Autodesk Inventor part; units mm, degrees
ref_plane "YZ Plane" through (0, 0, 0) normal (1, 0, 0) x (0, 1, 0)
ref_plane "XZ Plane" through (0, 0, 0) normal (0, 1, 0) x (-1, 0, 0)
ref_plane "XY Plane" through (0, 0, 0) normal (0, 0, 1) x (1, 0, 0)
sketch "Boceto1" plane through (0, 0, 0) normal (0, 0, 1) x (1, 0, 0)
  point P0 (0, 0)
sketch "Boceto2" plane through (0, 0, 0) normal (0, 0, 1) x (1, 0, 0)
  line L0 (0, 0) -> (0, 100)
  line L1 (30, 130) -> (30, 130)
  line L2 (60, 100) -> (60, 0)
  line L3 (60, 0) -> (0, 0)
  arc A0 (30, 130) -> (0, 100) centre (30, 100) ccw
  arc A1 (60, 100) -> (30, 130) centre (30, 100) ccw
  point P0 (0, 130)
  point P1 (60, 130)
  dimension "d1" = 30
  dimension "d2" = 100
  dimension "d3" = 60
extrude "Extrusión1" add sketch "Boceto2" along normal mid plane 25
sketch "Boceto9" plane through (0, 0, 12.5) normal (0, -1, 0) x (1, 0, 0)
  circle A0 centre (50, -12.5) radius 4
  line L0 (60, -25) -> (0, -25)
  circle A1 centre (10, -12.5) radius 4
  line L1 (0, -12.5) -> (60, -12.5) construction
  line L2 (60, 0) -> (60, -25) construction
  dimension "d52" = 8
  dimension "d88" = 10
  dimension "d89" = 10
hole "Agujero4" at (10, 0, 0) at (50, 0, 0) direction (0, 1, 0) diameter 8 depth 25
thread "Rosca3"
thread "Rosca4"
sketch "Boceto10" plane through (0, 0, 12.5) normal (0, 0, 1) x (1, 0, 0)
  circle A0 centre (30, 100) radius 11
  circle A1 centre (30, 100) radius 13.0125
  line L0 (60, 0) -> (60, 100)
  line L1 (0, 100) -> (0, 0)
  line L2 (40, 144.843) -> (20, 144.843)
  dimension "d64" = 22
  dimension "d65" = 30
  dimension "d68" = 26.025
  dimension "d90" = 100
extrude "Extrusión5" cut sketch "Boceto10" against normal through all contours A0
extrude "Extrusión6" cut sketch "Boceto10" against normal blind 9
sketch "Boceto12" plane through (0, 0, 12.5) normal (0, 0, 1) x (1, 0, 0)
  line L0 (5, 21.5) -> (15, 21.5)
  line L1 (17, 19.5) -> (17, 17)
  line L2 (15, 15) -> (5, 15)
  line L3 (3, 17) -> (3, 19.5)
  line L4 (45, 21.5) -> (55, 21.5)
  line L5 (57, 19.5) -> (57, 17)
  line L6 (55, 15) -> (45, 15)
  line L7 (43, 17) -> (43, 19.5)
  line L8 (0, 0) -> (60, 0)
  line L9 (10, 0) -> (10, 43.0314) construction
  line L10 (54, 0) -> (46, 0) construction
  line L11 (50, 0) -> (50, 39.0292) construction
  arc A0 (5, 21.5) -> (3, 19.5) centre (5, 19.5) ccw
  arc A1 (3, 17) -> (5, 15) centre (5, 17) ccw
  arc A2 (15, 15) -> (17, 17) centre (15, 17) ccw
  arc A3 (17, 19.5) -> (15, 21.5) centre (15, 19.5) ccw
  arc A4 (45, 21.5) -> (43, 19.5) centre (45, 19.5) ccw
  arc A5 (43, 17) -> (45, 15) centre (45, 17) ccw
  arc A6 (57, 19.5) -> (55, 21.5) centre (55, 19.5) ccw
  arc A7 (55, 15) -> (57, 17) centre (55, 17) ccw
  point P0 (17, 15)
  point P1 (17, 21.5)
  point P2 (3, 15)
  point P3 (43, 21.5)
  point P4 (57, 15)
  point P5 (43, 15)
  dimension "d91" = 14
  dimension "d92" = 14
  dimension "d93" = 6.5
  dimension "d94" = 15
  dimension "d95" = 40
  dimension "d96" = 7
  dimension "d97" = 7
  dimension "d98" = 2
  dimension "d99" = 2
  dimension "d100" = 2
  dimension "d101" = 2
  dimension "d102" = 2
  dimension "d103" = 2
  dimension "d104" = 2
  dimension "d105" = 2
extrude "Extrusión7" cut sketch "Boceto12" against normal blind 20
sketch "Boceto13" plane through (0, 0, 12.5) normal (0, 0, 1) x (1, 0, 0)
  circle A0 centre (30, 20) radius 6
  line L0 (0, 0) -> (60, 0) construction
  line L1 (30, 0) -> (30, 20) construction
  dimension "d108" = 20
  dimension "d109" = 12
extrude "Extrusión8" cut sketch "Boceto13" against normal through all
equation "\"Radio_pliegue\" = Grosor"
equation "\"Anchura_desahogo_plegado\" = Grosor"
equation "\"Profundidad_desahogo_plegado\" = 0.5 * Grosor"
equation "\"Tamaño_destalonado\" = 4 * Grosor"
equation "\"Remanente_mínimo\" = 2 * Grosor"
equation "\"Radiodetransición\" = Radio_pliegue"
equation "\"Tamaño_de_radio_de_Jacobi\" = Grosor"
equation "\"TamañoSeparación\" = Grosor"
properties part number "soporte_riel" material "Nilón 6/6"
For this review, take the finished solid that the model builds, in its own axes (mm). A direction names the side the tool comes from. Give positions to 0.01 mm unless a question says otherwise; leave off trailing zeros. Loops run counter-clockwise (first coordinate to the right, second up) from the corner with the lowest first, then second, coordinate; pieces in that order, holes last.
Item 1: Draft analysis for pull direction X (two halves, no side actions). For faces 1 (the flat face through (30, 0, 0)), 2 (the flat face through (50, 25, 0)), 3 (the flat face through (0, 49, 0)), state which applies: +X half, -X half, draft (parallel to the pull), parting line (faces both ways), or undercut.
Item 2: Take a section at D-D, the plane y = 98. State the section outline as (x, z) points, and give its area (3 significant figures).
Item 3: Take a section at C-C, the plane x = 21.5. State the section outline as (y, z) points.
Item 4: Tool access review of faces 4 (the cylindrical face through (13.905, 7.605, 0.867)), 5 (the flat face through (17, 18, 3)), 6 (the cylindrical face through (28.568, 110.906, -4.388)): name each direction out of +Z, -Z, +X, -X, +Y, -Y from which nothing blocks a thin tool from reaching the whole face with its end or side.
Item 5: For line 1 along X through (y, z) = (7.5, 0); line 2 along Y through (x, z) = (30, -7.25); line 3 along Y through (x, z) = (30, 8), list the stretches that pass through material, from the lowest coordinate up.
Item 6: Insertion check: pin 1 (2 mm diameter, centred on x = 22, z = 0.5, fed in from +Y); pin 2 (4 mm diameter, centred on y = 109, z = -2, fed in from +X); pin 3 (1 mm diameter, centred on x = 37, z = 7.5, fed in from +Y). Each pin has a flat end and moves straight along its axis. Give the tip position at first contact, or say it passes through.
Item 7: Take a section at B-B, the plane y = 8.5. State the section outline as (x, z) points.
Item 8: Take a section at A-A, the plane z = 8.75. State the section outline as (x, y) points (1 decimal).
Calculated:
1. face 1: draft
1. face 2: undercut
1. face 3: -X half
2. outline: (0, -12.5) - (19.18, -12.5) - (19.18, 3.5) - (17.14, 3.5) - (17.14, 12.5) - (0, 12.5) - close; (40.82, -12.5) - (60, -12.5) - (60, 12.5) - (42.86, 12.5) - (42.86, 3.5) - (40.82, 3.5) - close
2. area: 922 mm2
3. outline: (0, -12.5) - (93.02, -12.5) - (93.02, 3.5) - (90.15, 3.5) - (90.15, 12.5) - (0, 12.5) - close; (106.98, -12.5) - (128.77, -12.5) - (128.77, 12.5) - (109.85, 12.5) - (109.85, 3.5) - (106.98, 3.5) - close
4. face 4: -Y
4. face 5: +Z
4. face 6: +Z, -Z
5. line 1: x = 0 to 6, 14 to 46, 54 to 60
5. line 2: y = 0 to 14, 26 to 89, 111 to 130
5. line 3: y = 0 to 14, 26 to 86.99, 113.01 to 130
6. pin 1: stops at y = 129.17
6. pin 2: stops at x = 59.17
6. pin 3: stops at y = 129.29
7. outline: (0, -12.5) - (60, -12.5) - (60, 12.5) - (0, 12.5) - close; hole circle Ø8 at (10, 0); hole circle Ø8 at (50, 0)
8. outline: (0, 0) - (60, 0) - (60, 100) arc R30 ccw to (0, 100) - close; hole (3, 17) arc R2 ccw to (5, 15) - (15, 15) arc R2 ccw to (17, 17) - (17, 19.5) arc R2 ccw to (15, 21.5) - (5, 21.5) arc R2 ccw to (3, 19.5) - close; hole circle Ø26 at (30, 100); hole circle Ø12 at (30, 20); hole (43, 17) arc R2 ccw to (45, 15) - (55, 15) arc R2 ccw to (57, 17) - (57, 19.5) arc R2 ccw to (55, 21.5) - (45, 21.5) arc R2 ccw to (43, 19.5) - close
